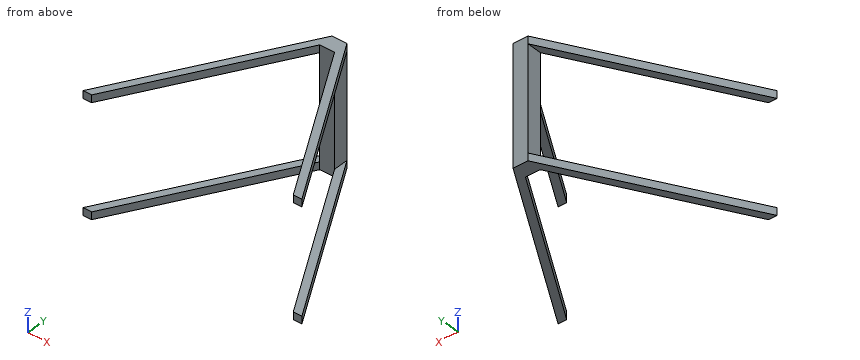
Autodesk Inventor part; units mm, degrees
ref_plane "YZ Plane" through (0, 0, 0) normal (1, 0, 0) x (0, 1, 0)
ref_plane "XZ Plane" through (0, 0, 0) normal (0, 1, 0) x (-1, 0, 0)
ref_plane "XY Plane" through (0, 0, 0) normal (0, 0, 1) x (1, 0, 0)
sketch "Sketch1" plane through (0, 0, 0) normal (0, 0, 1) x (1, 0, 0)
  point P0 (0, 0)
sketch "Sketch2" plane through (0, 0, 0) normal (0, 0, 1) x (1, 0, 0)
  line L0 (0, 650) -> (375.2777, 0)
  line L1 (409.9187, 0) -> (375.2777, 0)
  line L2 (409.9187, 0) -> (0, 710)
  line L3 (0, 650) -> (0, 710)
  point P0 (0, 0)
  dimension "d0" = 650
extrude "Extrusion1" add sketch "Sketch2" against normal blind 30
sketch "Sketch3" plane through (0, 0, 0) normal (0, 0, 1) x (1, 0, 0)
  line L0 (0, 650) -> (0, 710)
  line L1 (0, 650) -> (-60, 650)
  line L2 (-60, 650) -> (-60, 710)
  line L3 (-60, 710) -> (0, 710)
  line L4 (0, 710) -> (0, 650)
  line L5 (-60, 650) -> (-435.277, 0)
  line L6 (-60, 710) -> (-469.918, 0)
  line L7 (-469.918, 0) -> (-435.277, 0)
  point P0 (0, 0)
  dimension "d5" = 60
  dimension "d6" = 750.555
extrude "Extrusion2" add sketch "Sketch3" against normal blind 30 contours L5 L7 L6 L2
sketch "Sketch4" plane through (0, 0, 0) normal (0, 0, 1) x (1, 0, 0)
  line L0 (0, 710) -> (409.9187, 0)
  line L1 (-60, 650) -> (0, 650)
  line L2 (0, 650) -> (0, 710)
  line L3 (0, 710) -> (-60, 710)
  line L4 (-60, 710) -> (-60, 650)
  point P0 (0, 0)
extrude "Extrusion3" add sketch "Sketch4" against normal blind 60
sketch "Sketch5" plane through (0, 0, 0) normal (0, 0, 1) x (1, 0, 0)
  point P0 (0, 0)
sketch "Sketch6" plane through (0, 0, -60) normal (0, 0, -1) x (-1, 0, 0)
  line L0 (0, 710) -> (-409.9187, 0)
  line L1 (60, 650) -> (435.277, 0)
  line L2 (0, 710) -> (60, 710)
  line L3 (60, 710) -> (60, 650)
  line L4 (60, 650) -> (0, 650)
  line L5 (0, 650) -> (0, 710)
  point P0 (0, 0)
extrude "Extrusion4" add sketch "Sketch6" along normal blind 420
sketch "Sketch7" plane through (0, 0, -480) normal (0, 0, -1) x (-1, 0, 0)
  line L0 (60, 650) -> (435.277, 0)
  line L1 (60, 650) -> (435.277, 0)
  line L2 (469.918, 0) -> (60, 710)
  line L3 (435.277, 0) -> (469.918, 0)
  line L4 (469.918, 0) -> (60, 710)
  line L5 (60, 710) -> (60, 650)
  point P0 (0, 0)
extrude "Extrusion5" add sketch "Sketch7" against normal blind 30
sketch "Sketch8" plane through (0, 0, -480) normal (0, 0, -1) x (-1, 0, 0)
  line L0 (-375.2777, 0) -> (0, 650)
  line L1 (0, 650) -> (-375.2777, 0)
  line L2 (0, 710) -> (-409.9187, 0)
  line L3 (-375.2777, 0) -> (-409.9187, 0)
  line L4 (-409.9187, 0) -> (0, 710)
  line L5 (0, 710) -> (0, 650)
  point P0 (0, 0)
extrude "Extrusion6" add sketch "Sketch8" against normal blind 30
properties part number "stativ ide 1"
CAD build for the part. Positions are in the model's coordinates, mm. Give positions to 0.01 mm unless a question says otherwise; leave off trailing zeros. Write each loop counter-clockwise with the first axis right and the second up, starting at its lowest first coordinate (ties: lowest second). Pieces come first, ordered by that corner, then holes. Notation, with made-up numbers: (67.5, 66) - (124.5, 66) arc R13 cw to (124.5, 80) - close; hole circle Ø7 at (69, 1.25). An arc over 180 degrees is marked (long way). Put each result on its own line as item: value.
(1) Saw through at A-A (x = 338.5). List the corners of the cut face in (y, z).
Working result:
outline: (63.7, -480) - (123.7, -480) - (123.7, -450) - (63.7, -450) - close; (63.7, -30) - (123.7, -30) - (123.7, 0) - (63.7, 0) - close
(2) Saw through at D-D (x = -203). List the corners of the cut face in (y, z).
Working result:
outline: (402.32, -480) - (462.32, -480) - (462.32, -450) - (402.32, -450) - close; (402.32, -30) - (462.32, -30) - (462.32, 0) - (402.32, 0) - close
(3) Wall check: L1, parallel to Y at x = 72.5, z = -456. Give the ranges that are in metal, low to high.
Working result:
L1: 524.43 to 584.43
(4) Saw through at C-C (z = -63). List the corners of the cut face in (x, y).
Working result:
outline: (-60, 650) - (0, 650) - (0, 710) - (-60, 710) - close
(5) Saw through at B-B (y = 412). List the corners of the cut face in (x, z), then the cut area to 3 significant figures.
Working result:
outline: (-232.05, -480) - (-197.41, -480) - (-197.41, -450) - (-232.05, -450) - close; (-232.05, -30) - (-197.41, -30) - (-197.41, 0) - (-232.05, 0) - close; (137.41, -480) - (172.05, -480) - (172.05, -450) - (137.41, -450) - close; (137.41, -30) - (172.05, -30) - (172.05, 0) - (137.41, 0) - close
area: 4,160 mm^2
(6) Drop a flat-ended pin along its axis: pin 1 Ø18 at (x, z) = (-22, -146.5) entering from -Y. Give the stop position or say it passes through.
Working result:
pin 1: y = 650
